```python
from build123d import *

# Parameters (mm, degrees)
F2_R     = 45
F3_DEPTH = 80
F4_R     = 5
F5_DEPTH = 150.001


with BuildPart() as f1:
    # F0 (on Front) → F1 (revolve)
    with BuildSketch(Plane.XZ):
        Polygon((-52, 0), (0, 0), (0, 150), (-2, 150), (-7, 150), (-7, 138), (-16, 138), (-16, 126), (-25, 126), (-25, 114), (-34, 114), (-34, 102), (-43, 102), (-43, 90), (-52, 90), align=None)
    revolve(axis=Axis((0, 0, 75), (0, 0, 1)))

    # F2 (on Top) → F3 (cut)
    with BuildSketch(Plane.XY):
        Circle(F2_R)
    extrude(amount=F3_DEPTH, mode=Mode.SUBTRACT)

    # F4 (on Top) → F5 (cut, through all)
    with BuildSketch(Plane.XY):
        Circle(F4_R)
    extrude(amount=F5_DEPTH, mode=Mode.SUBTRACT)


solid = f1.part
```
For this review, take the finished solid that the model builds, in its own axes (mm). A direction names the side the tool comes from. Round coordinates to 2 decimals unless told otherwise and drop trailing zeros. Write each loop counter-clockwise with the first axis right and the second up, starting at its lowest first coordinate (ties: lowest second). Pieces come first, ordered by that corner, then holes. Notation, with made-up numbers: M -40,54.5 L -30,54.5 A29 cw -30,92.5 Z; hole C -20.5,43 d4. An arc over 180 degrees is marked long. One line per item, written item: value. Start each with the question number.
(1) Wall thickness on line 1 (Y direction, x = 0, z = 43); line 2 (X direction, y = 0, z = 132); line 3 (X direction, y = 0, z = 105.5): over which ranges is each line inside the solid? List them lowest first.
(2) Insertion check: pin 1 (6 mm diameter, centred on x = 17.5, y = 34.5, fed in from -Z); pin 2 (2 mm diameter, centred on x = -4, z = 130, fed in from -Y); pin 3 (6 mm diameter, centred on y = -37, z = 90, fed in from +X). Each pin has a flat end and moves straight along its axis. Give the tip position at first contact, or say it passes through.
(3) We need section C-C (z = 77). Give the boundary of the cut face in (x, y), and give its area (3 significant figures).
(4) Machinability: for faces 1 (the cylindrical face through (20.765, -39.923, 39.44)), 2 (the cylindrical face through (-23.846, -7.509, 119.916)), 3 (the flat face through (-2, -5, 150)), which of the approach directions +Z, -Z, +X, -X, +Y, -Y give a long, thin tool a straight path to every point of the face, cutting with its end or side? Answer none if there is none.
(5) The part is to be moulded in two halves that separate along Y. For faces 4 (the cylindrical face through (3.47, 15.62, 131.92)), 5 (the cylindrical face through (-1.08, -4.88, 114.51)), 6 (the flat face through (-1, -9, 80)), 7 (the flat face through (7, 3, 138)), say which applies: released by +Y, released by -Y, zero draft, split by the parting line, or undercut.
(6) We need section D-D (y = 18). Give the boundary of the cut face in (x, z).
Result:
1. line 1: -52 to -45, 45 to 52
1. line 2: -16 to -5, 5 to 16
1. line 3: -34 to -5, 5 to 34
2. pin 1: z = 80
2. pin 2: y = -15.72
2. pin 3: x = 39.34
3. outline: C 0,0 d104; hole C 0,0 d90
3. area: 2,130 mm²
4. face 1: -Z
4. face 2: +Z
4. face 3: +Z, +X, -X, +Y, -Y
5. face 4: split by the parting line
5. face 5: undercut
5. face 6: undercut
5. face 7: zero draft
6. outline: M -48.79,0 L -41.24,0 L -41.24,80 L 41.24,80 L 41.24,0 L 48.79,0 L 48.79,90 L 39.05,90 L 39.05,102 L 28.84,102 L 28.84,114 L 17.35,114 L 17.35,126 L -17.35,126 L -17.35,114 L -28.84,114 L -28.84,102 L -39.05,102 L -39.05,90 L -48.79,90 Z
